from build123d import *

# Parameters (mm, degrees)
F0_W     = 203.2
F0_H     = 101.6
F1_DEPTH = 25.4
F3_D     = 25.4
F4_R     = 38.1
F5_DEPTH = 25.4
F6_R     = 31.75
F7_DEPTH = 25.4
F8_R     = 38.1
F9_DEPTH = 25.4


with BuildPart() as f1:
    # F0 (on Front) → F1 (new body)
    with BuildSketch(Plane.XZ):
        Rectangle(F0_W, F0_H)
    extrude(amount=F1_DEPTH)

    # F3 (through all)
    with Locations(Plane.XZ.offset(25.4)):
        with Locations((-63.5, 31.75), (-63.5, -31.75), (63.5, -31.75), (63.5, 31.75)):
            Hole(F3_D / 2)



with BuildPart() as f5:
    # F4 (on face) → F5 (new body)
    with BuildSketch(Plane.XZ.offset(76.2)):
        Circle(F4_R)
    extrude(amount=F5_DEPTH)

    # F6 (on face) → F7 (join)
    with BuildSketch(Plane.XZ.offset(50.8)):
        Circle(F6_R)
    extrude(amount=F7_DEPTH)


with BuildPart() as f1_1:
    add(f1.part)

    add(f5.part)  # F9 merges F5
    # F8 (on face) → F9 (join)
    with BuildSketch(Plane.XZ.offset(25.4)):
        Circle(F8_R)
    extrude(amount=F9_DEPTH)


solid = f1_1.part
The model under review builds one solid part; all positions refer to its coordinate system, in mm. A direction names the side the tool comes from. Give positions to 0.01 mm unless a question says otherwise; leave off trailing zeros. Order: outer loops, then holes, each group sorted by start corner. A loop starts at its lowest first (then second) coordinate and runs counter-clockwise, first axis right, second up. Notation, with made-up numbers: (67, 19.25) -> (81, 19.25) arc R23 ccw to (81, 52.25) -> close; hole circle Ø4 at (52, -13). An arc over 180 degrees is marked (long way). Write item = value, one per line. Start each with the question number.
(1) Take a section at D-D (y = -95). Write out the cut boundary in (x, z), plus the area to 3 significant figures.
(2) For L1, parallel to Z at x = 63, y = -18; L2, parallel to X at y = -6, z = 31; L3, parallel to Y at x = 26.5, z = -18, list the stretches that pass through material, from the lowest coordinate up. Write a range as from..to.
(3) Take a section at B-B (z = 0). Write out the cut boundary in (x, y).
(4) Take a section at C-C (x = 0). Write out the cut boundary in (y, z).
(5) Take a section at A-A (x = -63.5). Write out the cut boundary in (y, z), plus the area to 3 significant figures.
(6) Tool access review of faces 1 (the cylindrical face through (-6.883, -63.322, -30.995)), 2 (the cylindrical face through (-30.235, -37.922, -23.183)), 3 (the flat face through (-1, -13, -50.8)): name each direction out of +Z, -Z, +X, -X, +Y, -Y from which nothing blocks a thin tool from reaching the whole face with its end or side.
(7) For pin 1 Ø6 at (x, z) = (65.5, 21) entering from -Y; pin 2 Ø6 at (y, z) = (-68.5, -11.5) entering from -X; pin 3 Ø2 at (y, z) = (-34, -5.5) entering from +X; pin 4 Ø15 at (x, z) = (-63.5, -31.75) entering from -Y, all flat-tipped, find the tip position at first contact; note any pin that passes through.
(8) Draft analysis for pull direction Y (two halves, no side actions). For faces 4 (the cylindrical face through (-30.235, -88.722, -23.183)), 5 (the flat face through (21, -25.4, 35)), 6 (the flat face through (-9, -76.2, 31)), 7 (the flat face through (-1, 0, 1)), state which applies: +Y half, -Y half, draft (parallel to the pull), parting line (faces both ways), or undercut.
Returned:
q1.outline = circle Ø76.2 at (0, 0)
q1.area = 4,560 mm²
q2.L1 = -50.8..-44.44, -19.06..19.06, 44.44..50.8
q2.L2 = -101.6..-76.18, -50.82..50.82, 76.18..101.6
q2.L3 = -101.6..-76.2, -50.8..0
q3.outline = (-101.6, -25.4) -> (-38.1, -25.4) -> (-38.1, -50.8) -> (-31.75, -50.8) -> (-31.75, -76.2) -> (-38.1, -76.2) -> (-38.1, -101.6) -> (38.1, -101.6) -> (38.1, -76.2) -> (31.75, -76.2) -> (31.75, -50.8) -> (38.1, -50.8) -> (38.1, -25.4) -> (101.6, -25.4) -> (101.6, 0) -> (-101.6, 0) -> close
q4.outline = (-101.6, -38.1) -> (-76.2, -38.1) -> (-76.2, -31.75) -> (-50.8, -31.75) -> (-50.8, -38.1) -> (-25.4, -38.1) -> (-25.4, -50.8) -> (0, -50.8) -> (0, 50.8) -> (-25.4, 50.8) -> (-25.4, 38.1) -> (-50.8, 38.1) -> (-50.8, 31.75) -> (-76.2, 31.75) -> (-76.2, 38.1) -> (-101.6, 38.1) -> close
q5.outline = (-25.4, -50.8) -> (0, -50.8) -> (0, -44.45) -> (-25.4, -44.45) -> close; (-25.4, -19.05) -> (0, -19.05) -> (0, 19.05) -> (-25.4, 19.05) -> close; (-25.4, 44.45) -> (0, 44.45) -> (0, 50.8) -> (-25.4, 50.8) -> close
q5.area = 1,290 mm²
q6.face_1 = none
q6.face_2 = -Y
q6.face_3 = -Z, +X, -X, +Y, -Y
q7.pin_1 = -25.4
q7.pin_2 = -30.59
q7.pin_3 = 37.83
q7.pin_4 = through
q8.face_4 = draft
q8.face_5 = -Y half
q8.face_6 = undercut
q8.face_7 = +Y half
